from build123d import *

# Parameters (mm, degrees)
F0_W     = 56
F0_H     = 63
F1_DEPTH = 2
F0_W_2   = 60
F0_H_2   = 65
F2_DEPTH = 16
F3_R     = 2
F4_DEPTH = 25


with BuildPart() as f1:
    # F0 (on Top) → F1 (new body)
    with BuildSketch(Plane.XY):
        with Locations((-30, -32.5)):
            Rectangle(F0_W, F0_H)
    extrude(amount=F1_DEPTH)

    # F0 (on Top) → F2 (join)
    with BuildSketch(Plane.XY):
        with Locations((-30, -32.5)):
            Rectangle(F0_W_2, F0_H_2)
        with Locations((-30, -32.5)):
            Rectangle(F0_W, F0_H, mode=Mode.SUBTRACT)
    extrude(amount=F2_DEPTH)

    # F3 (on face) → F4 (cut)
    with BuildSketch(Plane.XY.offset(2)):
        with Locations((-30, -20)):
            Circle(F3_R)
        with Locations((-30, -45)):
            Circle(F3_R)
    extrude(amount=-F4_DEPTH, mode=Mode.SUBTRACT)


solid = f1.part
Work out the finished part from the listing and answer in its coordinate system (mm). A direction names the side the tool comes from. Round coordinates to 2 decimals unless told otherwise and drop trailing zeros. Order: outer loops, then holes, each group sorted by start corner. A loop starts at its lowest first (then second) coordinate and runs counter-clockwise, first axis right, second up. Notation, with made-up numbers: M 76.5,58.5 L 127.5,58.5 A21 ccw 127.5,94.5 Z; hole C 7,-25.5 d3. An arc over 180 degrees is marked long. Put each result on its own line as item: value. Start each with the question number.
Q1. Straight lines are drawn through the part: L1, parallel to Y at x = -30, z = 1.25; L2, parallel to X at y = -55.5, z = 4.25; L3, parallel to Y at x = -39, z = 12.5. For each, find the intervals that lie inside material, in ascending order. Write a range as [from, to].
Q2. Flat-ended cylindrical pins translate along their axes: pin 1 (4 mm diameter, centred on y = -42, z = 6, fed in from +X); pin 2 (5 mm diameter, centred on x = -42, y = -20.5, fed in from +Z). Find the tip coordinate at first contact, or state that the pin passes through.
Q3. A tool of negligible diameter and unlimited length cuts with its end or side. For faces 1 (the flat face through (-30, -32, 2)), 2 (the flat face through (-30, 0, 8)), from which of +Z, -Z, +X, -X, +Y, -Y can it reach the whole face along a straight path? Write none if from no direction.
Q4. Section D-D, the plane y = -59 is taken. Write down the section's boundary in (x, z), and give its area (3 significant figures).
Q5. Section B-B, the plane x = -30 is taken. Write down the section's boundary in (y, z).
Q6. For a pull along X with two mould halves and no side action, classify faces 3 (the flat face through (-60, -33, 8)), 4 (the cylindrical face through (-28.092, -19.399, 1.014)), 5 (the flat face through (0, -33, 8)) as pulls with the +X half, pulls with the -X half, needs draft (parallel to the pull), parting line crosses it, or undercut.
Q7. Section A-A, the plane y = -45 is taken. Write down the section's boundary in (x, z).
Q8. Section C-C, the plane z = 10 is taken. Write down the section's boundary in (x, y).
Findings below:
1. L1: y = [-65, -47], [-43, -22], [-18, 0]
1. L2: x = [-60, -58], [-2, 0]
1. L3: y = [-65, -64], [-1, 0]
2. pin 1: stops at x = 0
2. pin 2: stops at z = 2
3. face 1: +Z
3. face 2: +Z, -Z, +X, -X, +Y
4. outline: M -60,0 L 0,0 L 0,16 L -2,16 L -2,2 L -58,2 L -58,16 L -60,16 Z
4. area: 176 mm^2
5. outline: M -65,0 L -47,0 L -47,2 L -64,2 L -64,16 L -65,16 Z; M -43,0 L -22,0 L -22,2 L -43,2 Z; M -18,0 L 0,0 L 0,16 L -1,16 L -1,2 L -18,2 Z
6. face 3: pulls with the -X half
6. face 4: undercut
6. face 5: pulls with the +X half
7. outline: M -60,0 L -32,0 L -32,2 L -58,2 L -58,16 L -60,16 Z; M -28,0 L 0,0 L 0,16 L -2,16 L -2,2 L -28,2 Z
8. outline: M -60,-65 L 0,-65 L 0,0 L -60,0 Z; hole M -58,-64 L -2,-64 L -2,-1 L -58,-1 Z
